For this review, take the finished solid that the model builds, in its own axes (mm). Face numbers are marked on the shaded views. A direction names the side the tool comes from. Coordinates: 2 decimals unless noted, no trailing zeros. Order: outer loops, then holes, each group sorted by start corner. A loop starts at its lowest first (then second) coordinate and runs counter-clockwise, first axis right, second up. Notation, with made-up numbers: (9.5, -32) -> (34.5, -32) arc R22 ccw to (34.5, -16) -> close; hole circle Ø7 at (-9, 60.5). An arc over 180 degrees is marked (long way). Return JSON: item names as keys, results as strings. Group by question number.
Item 1: Take a section at B-B (y = 8). Count the separate pieces of the cut face and the enclosed holes in it, then the cut area to 3 significant figures.
Item 2: Take a section at D-D (z = -27.5). Write out the cut boundary in (x, y), then the cut area to 3 significant figures.
Item 3: Take a section at A-A (x = 24.13). Write out the cut boundary in (y, z).
Item 4: Machinability: for the marked faces 1, 2 and 3, which of the approach directions +Z, -Z, +X, -X, +Y, -Y give a long, thin tool a straight path to every point of the face, cutting with its end or side? Answer none if there is none.
Item 5: Draft analysis for pull direction X (two halves, no side actions). For the marked faces 4, 5 and 6, state which applies: +X half, -X half, draft (parallel to the pull), parting line (faces both ways), or undercut.
Item 6: Take a section at C-C (x = -3.5). Write out the cut boundary in (y, z), then the cut area to 3 significant figures.
Item 7: Insertion check: pin 1 (3 mm diameter, centred on x = 25.5, y = 6, fed in from -Z); pin 2 (1.5 mm diameter, centred on y = 7.5, z = 6, fed in from -X); pin 3 (12 mm diameter, centred on x = 24.5, z = -3.5, fed in from +Y). Each pin has a flat end and moves straight along its axis. Give the tip position at first contact, or say it passes through.
Item 8: For line 1 along X through (y, z) = (6.75, 7.5); line 2 along Z through (x, y) = (-31, -4.25); line 3 along X through (y, z) = (1.6, -12.05), list the stretches that pass through material, from the lowest coordinate up.
```python
from build123d import *

# Parameters (mm, degrees)
SKETCH1_W           = 70
SKETCH1_H           = 82.5
BOSS_EXTRUDE1_DEPTH = 2
SKETCH2_R           = 1.5875
CUT_EXTRUDE1_DEPTH  = 55.134670037
FILLET1_R           = 2.54
SKETCH2_3_W         = 5.08
SKETCH2_3_H         = 48.26
SKETCH2_3_W_2       = 2.54
SKETCH2_3_H_2       = 20.32
SKETCH2_3_H_3       = 15.24
SKETCH2_3_H_4       = 5.08
SKETCH2_3_H_5       = 25.4
BOSS_EXTRUDE2_DEPTH = 8.500000018
SKETCH4_W           = 8
SKETCH4_H           = 9.13
BOSS_EXTRUDE3_DEPTH = 4
SKETCH4_3_W         = 6
SKETCH4_3_H         = 6
BOSS_EXTRUDE4_DEPTH = 3.8
SKETCH5_R           = 2.25
BOSS_EXTRUDE5_DEPTH = 6.6
SKETCH6_W           = 10
SKETCH6_H           = 10
BOSS_EXTRUDE6_DEPTH = 1.4
CHAMFER1_SIZE       = 1.27


with BuildPart() as part:
    # Sketch1 → Boss-Extrude1 (new body)
    with BuildSketch(Plane(origin=(0, 0, 0), x_dir=(1, 0, 0), z_dir=(0, 1, 0))):
        Rectangle(SKETCH1_W, SKETCH1_H)
    extrude(amount=BOSS_EXTRUDE1_DEPTH)

    # Sketch2 → Cut-Extrude1 (cut, through all)
    with BuildSketch(Plane(origin=(0, 2, 0), x_dir=(1, 0, 0), z_dir=(0, 1, 0))):
        with Locations(Location((8.89, -38.75, 0), (0, 0, 270))):
            Circle(SKETCH2_R)
        with Locations(Location((24.13, 12.05, 0), (0, 0, 270))):
            Circle(SKETCH2_R)
        with Locations(Location((-24.13, 13.32, 0), (0, 0, 270))):
            Circle(SKETCH2_R)
        Polygon((-35, -41.25), (-35, -39.25), (-24.13, -39.25), (-22.13, -41.25), align=None)
        Polygon((35, -39.25), (12.87, -39.25), (10.87, -41.25), (35, -41.25), align=None)
    extrude(amount=-CUT_EXTRUDE1_DEPTH, mode=Mode.SUBTRACT)

    # Fillet1
    fillet1_edges = [part.edges().sort_by_distance(p)[0] for p in [
        (35, 1, 39.25),
        (-35, 1, 39.25),
        (-35, 1, -41.25),
        (35, 1, -41.25),
    ]]
    fillet(fillet1_edges, radius=FILLET1_R)

    # Sketch2_3 → Boss-Extrude2 (add, symmetric)
    with BuildSketch(Plane(origin=(0, 2, 0), x_dir=(1, 0, 0), z_dir=(0, 1, 0))):
        with Locations((-30.48, -13.35)):
            Rectangle(SKETCH2_3_W, SKETCH2_3_H)
        with Locations((-24.13, -9.54)):
            Rectangle(SKETCH2_3_W_2, SKETCH2_3_H_2)
        with Locations((-24.13, -29.86)):
            Rectangle(SKETCH2_3_W_2, SKETCH2_3_H_3)
        with Locations((30.48, -13.35)):
            Rectangle(SKETCH2_3_W, SKETCH2_3_H)
        with Locations((31.75, 36.18)):
            Rectangle(SKETCH2_3_W_2, SKETCH2_3_H_4)
        with Locations((-31.75, 36.18)):
            Rectangle(SKETCH2_3_W_2, SKETCH2_3_H_4)
        with Locations((24.13, -2.94)):
            Rectangle(SKETCH2_3_W_2, SKETCH2_3_H_5)
        with Locations((24.13, -27.32)):
            Rectangle(SKETCH2_3_W_2, SKETCH2_3_H_2)
    extrude(amount=BOSS_EXTRUDE2_DEPTH, both=True)

    # Sketch4 → Boss-Extrude3 (add)
    with BuildSketch(Plane(origin=(0, 2, 0), x_dir=(1, 0, 0), z_dir=(0, 1, 0))):
        with Locations((11.8, 38.145)):
            Rectangle(SKETCH4_W, SKETCH4_H)
    extrude(amount=BOSS_EXTRUDE3_DEPTH)

    # Sketch4_3 → Boss-Extrude4 (add)
    with BuildSketch(Plane(origin=(0, 2, 0), x_dir=(1, 0, 0), z_dir=(0, 1, 0))):
        with Locations((-8, 13.25)):
            Rectangle(SKETCH4_3_W, SKETCH4_3_H)
        with Locations((8.4, 13.25)):
            Rectangle(SKETCH4_3_W, SKETCH4_3_H)
    extrude(amount=BOSS_EXTRUDE4_DEPTH)

    # Sketch5 → Boss-Extrude5 (add)
    with BuildSketch(Plane(origin=(0, 5.8, 0), x_dir=(1, 0, 0), z_dir=(0, 1, 0))):
        with Locations(Location((-8, 13.25, 0), (0, 0, 270))):
            Circle(SKETCH5_R)
        with Locations(Location((8.4, 13.25, 0), (0, 0, 270))):
            Circle(SKETCH5_R)
    extrude(amount=BOSS_EXTRUDE5_DEPTH)

    # Sketch6 → Boss-Extrude6 (add)
    with BuildSketch(Plane(origin=(0, 2, 0), x_dir=(1, 0, 0), z_dir=(0, 1, 0))):
        with Locations((-2.6, -17.65)):
            Rectangle(SKETCH6_W, SKETCH6_H)
    extrude(amount=BOSS_EXTRUDE6_DEPTH)

    # Chamfer1
    chamfer1_edges = [part.edges().sort_by_distance(p)[0] for p in [
        (2.4, 2.7, 22.65),
        (2.4, 2.7, 12.65),
        (-7.6, 2.7, 12.65),
        (-7.6, 2.7, 22.65),
    ]]
    chamfer(chamfer1_edges, length=CHAMFER1_SIZE)


solid = part.part
```
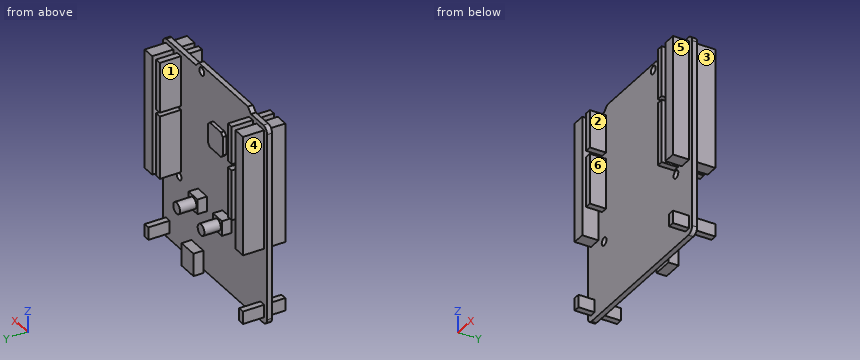
Findings below:
{
 "1": {"separate pieces": "10", "enclosed holes": "0", "area": "754 mm2"},
 "2": {"outline": "(-35, 0) -> (35, 0) -> (35, 2) -> (-35, 2) -> close", "area": "140 mm2"},
 "3": {"outline": "(-6.5, -9.76) -> (0, -9.76) -> (0, -10.46) -> (2, -10.46) -> (2, -9.76) -> (10.5, -9.76) -> (10.5, 15.64) -> (2, 15.64) -> (2, 17.16) -> (10.5, 17.16) -> (10.5, 37.48) -> (2, 37.48) -> (2, 39.25) -> (0, 39.25) -> (0, 37.48) -> (-6.5, 37.48) -> (-6.5, 17.16) -> (0, 17.16) -> (0, 15.64) -> (-6.5, 15.64) -> close; (0, -41.25) -> (2, -41.25) -> (2, -13.64) -> (0, -13.64) -> close"},
 "4": {"face 1": "+Z, -Z, +Y", "face 2": "+Z, -Z, -Y", "face 3": "+Z, -Z, +X, +Y"},
 "5": {"face 4": "-X half", "face 5": "+X half", "face 6": "undercut"},
 "6": {"outline": "(0, -41.25) -> (2, -41.25) -> (2, 12.65) -> (3.4, 12.65) -> (3.4, 22.65) -> (2, 22.65) -> (2, 41.25) -> (0, 41.25) -> close", "area": "179 mm2"},
 "7": {"pin 1": "stops at z = -9.76", "pin 2": "stops at x = -33.02", "pin 3": "stops at y = 10.5"},
 "8": {"line 1": "x = -33.02 to -27.94, -25.4 to -22.86, 22.86 to 25.4, 27.94 to 33.02", "line 2": "z = -38.72 to -33.64, -10.78 to 37.48", "line 3": "x = -35 to -25.08, -23.18 to 22.54, 25.72 to 35"}
}
